Check sheet for the modelled part. Datum: model origin and axes. Units: mm. A direction names the side the tool comes from. Give positions to 0.01 mm unless a question says otherwise; leave off trailing zeros. Order: outer loops, then holes, each group sorted by start corner. A loop starts at its lowest first (then second) coordinate and runs counter-clockwise, first axis right, second up.
```python
from build123d import *

# Parameters (mm, degrees)
F1_DEPTH = 28.575
F2_SIZE2 = 15.875
F2_SIZE  = 50.8


with BuildPart() as f1:
    # F0 (on Top) → F1 (new body)
    with BuildSketch(Plane.XY):
        with BuildLine():
            Line((228.6, 457.2), (-685.8, 457.2))
            Line((-685.8, 457.2), (-685.8, -457.2))
            Line((-685.8, -457.2), (228.6, -457.2))
            ThreePointArc((228.6, -457.2), (551.8892203585, -323.2892203585), (685.8, 0))
            ThreePointArc((685.8, 0), (551.8892203585, 323.2892203585), (228.6, 457.2))
        make_face()
        Polygon((152.4, 123.825), (152.4, 0), (152.4, -123.825), (101.6, -123.825), (101.6, 123.825), align=None, mode=Mode.SUBTRACT)
    extrude(amount=F1_DEPTH)

    # F2
    f2_edges = [f1.edges().sort_by_distance(p)[0] for p in [
        (-228.6, 457.2, 0),
        (685.8, 0, 0),
        (-228.6, -457.2, 0),
    ]]
    f2_side = f1.faces().sort_by_distance((-46.847704, 0, 0))[0]
    chamfer(f2_edges, length=F2_SIZE, length2=F2_SIZE2, reference=f2_side)


solid = f1.part
```
Q1. Sectioned sample at C-C, the plane z = 8. Record the cut outline in (x, y) (3 decimals).
Q2. Material ranges on line 1 (Y direction, x = 109, z = 16) (3 decimals); line 2 (X direction, y = 73, z = 22.5); line 3 (X direction, y = 97, z = 20.75), recorded low to high.
Q3. Go/stop test with flat-tipped pins: P1, Ø6, axis at y = 247, z = 19, coming from the +X side; P2, Ø8, axis at y = 348, z = 17, coming from the +X side. Record where each tip stops, or that it passes through.
Q4. Sectioned sample at A-A, the plane y = 0. Record the cut outline in (x, z) (3 decimals).
Q5. Draft check along X on faces 3 (the flat face through (-10, 6, 28.575)), 4 (the flat face through (127, 123.825, 14)), 5 (the flat face through (-685.8, 6, 14)). Enter one of: pulls with the +X half, pulls with the -X half, needs draft (parallel to the pull), parting line crosses it, or undercut.
Q6. Tool access check on faces 1 (the flat face through (101.6, -2, 14)), 2 (the flat face through (-222, 432, 8)). Record the directions out of +Z, -Z, +X, -X, +Y, -Y that give a thin tool (end or side, any length) a straight path to the whole face; none if there is none.
Q7. Sectioned sample at D-D, the plane x = -103. Record the cut outline in (y, z) (3 decimals), plus the area to 3 significant figures.
Q8. Sectioned sample at B-B, the plane x = 117.5. Record the cut outline in (y, z) (3 decimals).
Filled in:
1. outline: (-685.8, -432) - (228.6, -432) arc R432 ccw to (228.6, 432) - (-685.8, 432) - close; hole (101.6, -123.825) - (152.4, -123.825) - (152.4, 123.825) - (101.6, 123.825) - close
2. line 1: y = -457.2 to -123.825, 123.825 to 457.2
2. line 2: x = -685.8 to 101.6, 152.4 to 679.93
2. line 3: x = -685.8 to 101.6, 152.4 to 675.39
3. P1: stops at x = 615.25
3. P2: stops at x = 529.76
4. outline: (-685.8, 0) - (101.6, 0) - (101.6, 28.575) - (-685.8, 28.575) - close; (152.4, 0) - (635, 0) - (685.8, 15.875) - (685.8, 28.575) - (152.4, 28.575) - close
5. face 3: needs draft
5. face 4: undercut
5. face 5: pulls with the -X half
6. face 1: +Z, -Z
6. face 2: -Z, +X, -X, +Y
7. outline: (-457.2, 15.875) - (-406.4, 0) - (406.4, 0) - (457.2, 15.875) - (457.2, 28.575) - (-457.2, 28.575) - close
7. area: 25,300 mm2
8. outline: (-457.2, 15.875) - (-406.4, 0) - (-123.825, 0) - (-123.825, 28.575) - (-457.2, 28.575) - close; (123.825, 0) - (406.4, 0) - (457.2, 15.875) - (457.2, 28.575) - (123.825, 28.575) - close
